Geometry: final body of the model. Coordinates: model frame, mm. A direction names the side the tool comes from. Round coordinates to 2 decimals unless told otherwise and drop trailing zeros. Write each loop counter-clockwise with the first axis right and the second up, starting at its lowest first coordinate (ties: lowest second). Pieces come first, ordered by that corner, then holes. Notation, with made-up numbers: (31, -38) -> (55, -38) arc R22 ccw to (55, -5) -> close; hole circle Ø11 at (88, 6). An arc over 180 degrees is marked (long way). Use one line per item in the form item = value. Start each with the question number.
1. Line query: L1, parallel to Y at x = 31.5, z = 101; L2, parallel to X at y = 45.5, z = 123.5. Output: solid intervals per line, ascending.
2. Reachability of faces 1 (the face through (0, 25, 100)), 2 (the face through (26, 6.35, 100)) from +Z, -Z, +X, -X, +Y, -Y: full face, straight path, thin tool, end or side. Return the list, or none.
3. Pin query (flat end, axial travel): pin 1 Ø3 at (y, z) = (10, 140.5) entering from +X; pin 2 Ø2 at (y, z) = (31.5, 126) entering from +X; pin 3 Ø11.5 at (x, z) = (26, 144) entering from +Y. Return the tip coordinate at first contact, or that it passes through.
4. Cut plane B-B, the plane x = 16. Return the cut outline in (y, z), plus the area to 3 significant figures.
5. Cut plane A-A, the plane z = 116. Return the cut outline in (x, y).
```python
from build123d import *

# Parameters (mm, degrees)
BOSS_EXTRUDE1_DEPTH = 203.2


with BuildPart() as part:
    # Sketch1 → Boss-Extrude1 (new body)
    with BuildSketch(Plane.XY):
        with BuildLine():
            ThreePointArc((1.27, 50.342576275), (4.862102448, 48.854678723), (6.35, 45.262576275))
            Line((6.35, 45.262576275), (6.35, 6.35))
            Line((6.35, 6.35), (45.262576275, 6.35))
            ThreePointArc((45.262576275, 6.35), (48.854678723, 4.862102448), (50.342576275, 1.27))
            Line((50.342576275, 1.27), (50.342576275, 0))
            Line((50.342576275, 0), (0, 0))
            Line((0, 0), (0, 50.342576275))
            Line((0, 50.342576275), (1.27, 50.342576275))
        make_face()
    extrude(amount=BOSS_EXTRUDE1_DEPTH)


solid = part.part
```
Outcome:
q1.L1 = 0 to 6.35
q1.L2 = 0 to 6.34
q2.face_1 = +Z, -Z, -X, +Y, -Y
q2.face_2 = +Z, -Z, +X, +Y
q3.pin_1 = 6.35
q3.pin_2 = 6.35
q3.pin_3 = 6.35
q4.outline = (0, 0) -> (6.35, 0) -> (6.35, 203.2) -> (0, 203.2) -> close
q4.area = 1,290 mm^2
q5.outline = (0, 0) -> (50.34, 0) -> (50.34, 1.27) arc R5.08 ccw to (45.26, 6.35) -> (6.35, 6.35) -> (6.35, 45.26) arc R5.08 ccw to (1.27, 50.34) -> (0, 50.34) -> close
